Autodesk Inventor part; units mm, degrees
ref_plane "YZ Plane" through (0, 0, 0) normal (1, 0, 0) x (0, 1, 0)
ref_plane "XZ Plane" through (0, 0, 0) normal (0, 1, 0) x (-1, 0, 0)
ref_plane "XY Plane" through (0, 0, 0) normal (0, 0, 1) x (1, 0, 0)
sketch "Sketch1" plane through (0, 0, 0) normal (0, 1, 0) x (-1, 0, 0)
  line L0 (0, 0) -> (0, -270.8) construction
  line L1 (0, -270.8) -> (47.15, -270.8) construction
  line L2 (0, -120.8) -> (10.5, -120.8) construction
  line L3 (0, -20.8) -> (9.5, -20.8) construction
  line L4 (0, -15.3) -> (12.6, -15.3) construction
  line L5 (0, 0) -> (10.5, 0) construction
  line L6 (10.5, 0) -> (10.5, -15.3)
  line L7 (10.5, -15.3) -> (12.6, -15.3)
  line L8 (12.6, -15.3) -> (9.5, -20.8)
  line L9 (10.5, -120.8) -> (9.5, -20.8)
  arc A0 (10.5, -120.8) -> (47.15, -270.8) centre (349.6639, -117.4084) ccw
  arc A1 (8.9999, -120.8) -> (45.4691, -270.8) centre (349.6639, -117.4084) ccw
  line L10 (8.9999, -120.8) -> (7.7919, 0)
  line L11 (10.5, 0) -> (7.7919, 0)
  arc A2 (45.4691, -270.8) -> (47.15, -270.8) centre (46.3096, -270.3762) ccw
  dimension "d0" = 15.3
  dimension "d1" = 5.5
  dimension "d2" = 100
  dimension "d3" = 150
  dimension "d4" = 47.15
  dimension "d5" = 10.5
  dimension "d6" = 9.5
  dimension "d7" = 12.6
  dimension "d8" = 10.5
  dimension "d9" = 1.5
revolve "Revolution1" add sketch "Sketch1" angle 360 about axis through (0, 0, 0) along (0, 0, -1)
thread "Thread1"
equation "\"d0\" = Mount_Length"
equation "\"d1\" = Mount_Flange_Length"
equation "\"d2\" = Transition_Length"
equation "\"d3\" = Flare_Length"
equation "\"d4\" = Flare_Diameter"
equation "\"d5\" = Transition_Diameter"
equation "\"d6\" = Tail_Diameter"
equation "\"d7\" = Mount_Flange_Diameter"
equation "\"d8\" = Mount_Diameter"
equation "\"d9\" = Bell_Thickness"
equation "\"Transition_Length\" = 100"
properties part number "Horn_B" material "Steel, Cast"
Work out the finished part from the listing and answer in its coordinate system (mm). A direction names the side the tool comes from. Round coordinates to 2 decimals unless told otherwise and drop trailing zeros. Write each loop counter-clockwise with the first axis right and the second up, starting at its lowest first coordinate (ties: lowest second). Pieces come first, ordered by that corner, then holes.
1) A cutting plane is placed at B-B on z = -33. Determine the outline of the cut face in (x, y), and give its area (3 significant figures).
2) Flat-ended cylindrical pins translate along their axes: P1, Ø6, axis at y = 9.5, z = -188.5, coming from the +X side; P2, Ø2, axis at y = -6, z = -201, coming from the -X side; P3, Ø5, axis at y = -22.5, z = -225, coming from the -X side. Find the tip coordinate at first contact, or state that the pin passes through.
3) Consider probe 1 along X at (y, z) = (0, -118.5); probe 2 along X at (y, z) = (6.5, -201.5); probe 3 along Y at (x, z) = (-1.5, -156). Determine where each line is inside the solid, lowest interval first.
4) Which of the six approach directions +Z, -Z, +X, -X, +Y, -Y give full straight-line access (tool end or side, diameter ignored) to faces 1 (the face through (-10, 3.2, -7.8)), 2 (the face through (7.94, -6.09, -71.5))?
5) Determine the mould class of faces 3 (the face through (6.67, -5.11, -61.25)), 4 (the face through (0, 8, 0)), 5 (the face through (1.26, -9.61, -20.46)) for opening direction Z: pulls with the +Z half, pulls with the -Z half, needs draft (parallel to the pull), parting line crosses it, or undercut.
6) A cutting plane is placed at A-A on z = -148.5. Determine the outline of the cut face in (x, y), and give its area (3 significant figures).
Entries:
1. outline: circle Ø19.24 at (0, 0); hole circle Ø16.24 at (0, 0)
1. area: 83.6 mm2
2. P1: stops at x = 16.99
2. P2: stops at x = -20.45
2. P3: stops at x = -19.86
3. probe 1: x = -10.48 to -8.98, 8.98 to 10.48
3. probe 2: x = -20.05 to -18.41, 18.41 to 20.05
3. probe 3: y = -12.6 to -11.07, 11.07 to 12.6
4. face 1: +Z
4. face 2: none
5. face 3: pulls with the -Z half
5. face 4: pulls with the +Z half
5. face 5: undercut
6. outline: circle Ø23.82 at (0, 0); hole circle Ø20.81 at (0, 0)
6. area: 106 mm2
